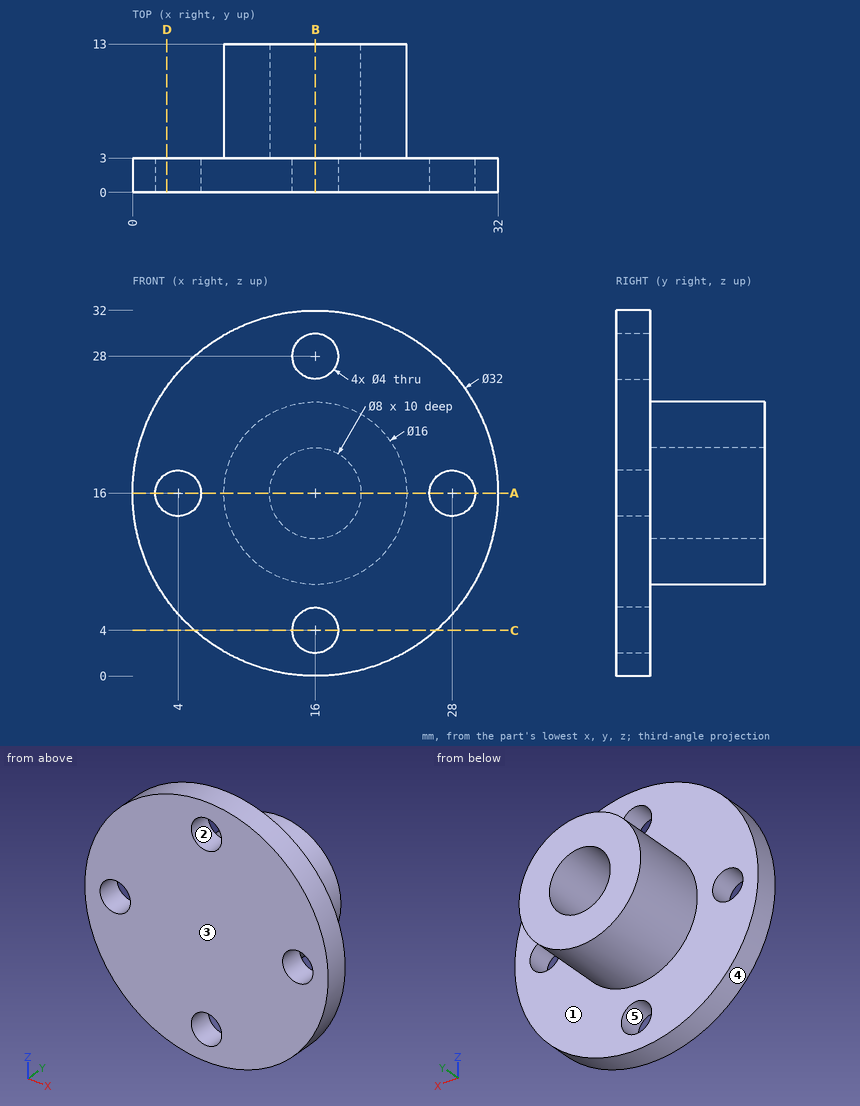
Answer from the drawing. Dimensions are ordinates in mm from the lowest x, y and z of the part. A direction names the side the tool comes from. Give positions to 0.01 mm unless a question says otherwise; leave off trailing zeros. Order: outer loops, then holes, each group sorted by start corner. A loop starts at its lowest first (then second) coordinate and runs counter-clockwise, first axis right, second up. Notation, with made-up numbers: (32.5, -5.5) - (66.5, -5.5) arc R23 ccw to (66.5, 20.5) - close; hole circle Ø8 at (-5.5, 55). An arc over 180 degrees is marked (long way). One line per item, written item: value. Start each with the question number.
1) Find the intervals of material crossed by L1, parallel to Z at x = 16, y = 2; L2, parallel to X at y = 6.5, z = 16, in increasing order.
2) A cutting plane is placed at D-D on x = 3. Give the vertices of the cut face in (y, z), then the cut area to 3 significant figures.
3) A cutting plane is placed at B-B on x = 16. Give the vertices of the cut face in (y, z).
4) The mould has two halves that part along X. Classify the marked faces 3, 4 and 5: released by +X, released by -X, zero draft, split by the parting line, or undercut.
5) A cutting plane is placed at C-C on z = 4. Give the vertices of the cut face in (x, y).
6) A tool of negligible diameter and unlimited length cuts with its end or side. For the marked faces 1 and 2, from which of +Z, -Z, +X, -X, +Y, -Y can it reach the whole face along a straight path? Write none if from no direction.
7) Given pin 1 Ø3 at (y, z) = (10, 14.5) entering from +X; pin 2 Ø3 at (x, z) = (16, 28) entering from +Y; pin 3 Ø5 at (x, z) = (16, 16) entering from +Y; pin 4 Ø12 at (x, z) = (28.5, 9) entering from -Y, each flat-ended and moving along its own axis, determine where each tip first touches the part or whether it passes through.
8) A cutting plane is placed at A-A on z = 16. Give the vertices of the cut face in (x, y), then the cut area to 3 significant figures.
Answer sheet:
1. L1: z = 0 to 2, 6 to 26, 30 to 32
1. L2: x = 8 to 12, 20 to 24
2. outline: (0, 6.67) - (3, 6.67) - (3, 14.27) - (0, 14.27) - close; (0, 17.73) - (3, 17.73) - (3, 25.33) - (0, 25.33) - close
2. area: 45.6 mm2
3. outline: (0, 0) - (3, 0) - (3, 2) - (0, 2) - close; (0, 6) - (3, 6) - (3, 8) - (13, 8) - (13, 12) - (3, 12) - (3, 20) - (13, 20) - (13, 24) - (3, 24) - (3, 26) - (0, 26) - close; (0, 30) - (3, 30) - (3, 32) - (0, 32) - close
4. face 3: zero draft
4. face 4: split by the parting line
4. face 5: undercut
5. outline: (5.42, 0) - (14, 0) - (14, 3) - (5.42, 3) - close; (18, 0) - (26.58, 0) - (26.58, 3) - (18, 3) - close
6. face 1: +Y
6. face 2: +Y, -Y
7. pin 1: stops at x = 24
7. pin 2: passes through
7. pin 3: stops at y = 3
7. pin 4: stops at y = 0
8. outline: (0, 0) - (2, 0) - (2, 3) - (0, 3) - close; (6, 0) - (26, 0) - (26, 3) - (24, 3) - (24, 13) - (20, 13) - (20, 3) - (12, 3) - (12, 13) - (8, 13) - (8, 3) - (6, 3) - close; (30, 0) - (32, 0) - (32, 3) - (30, 3) - close
8. area: 152 mm2
